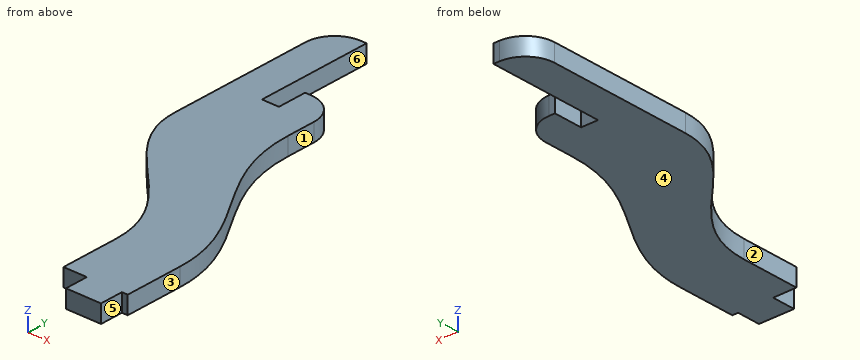
```python
from build123d import *

# Parameters (mm, degrees)
SKETCH1_W           = 6
SKETCH1_H           = 4
BOSS_EXTRUDE1_DEPTH = 3
FILLET1_R           = 5


with BuildPart() as part:
    # Sketch1 → Boss-Extrude1 (new body)
    with BuildSketch(Plane.XY):
        with BuildLine():
            Line((0, 0), (-11, 0))
            Line((-11, 0), (-11, 10))
            add(Edge.make_bspline(
                [(-11, 10), (-11, 23.756315473), (-27.75, 27.611609377), (-27.75, 40)],
                knots=[0, 0, 0, 0, 1, 1, 1, 1], degree=3))
            Line((-27.75, 40), (-27.75, 70))
            Line((-27.75, 70), (-21.75, 70))
            Line((-21.75, 70), (-21.75, 50))
            Line((-21.75, 50), (-18.85, 50))
            Line((-18.85, 50), (-18.85, 55))
            Line((-18.85, 55), (-12.85, 55))
            Line((-12.85, 55), (-12.85, 45))
            add(Edge.make_bspline(
                [(-12.85, 45), (-12.85, 29.868343374), (0, 23.949472312), (0, 10)],
                knots=[0, 0, 0, 0, 1, 1, 1, 1], degree=3))
            Line((0, 10), (0, 0))
        make_face()
        with Locations((-4, -2)):
            Rectangle(SKETCH1_W, SKETCH1_H)
    extrude(amount=BOSS_EXTRUDE1_DEPTH)

    # Fillet1
    fillet1_edges = [part.edges().sort_by_distance(p)[0] for p in [
        (-27.75, 70, 1.5),
        (-12.85, 55, 1.5),
    ]]
    fillet(fillet1_edges, radius=FILLET1_R)


solid = part.part
```
Build history of the part. All positions in model axes, mm. Face numbers are marked on the shaded views. A direction names the side the tool comes from. Round coordinates to 2 decimals unless told otherwise and drop trailing zeros. Write each loop counter-clockwise with the first axis right and the second up, starting at its lowest first coordinate (ties: lowest second). Pieces come first, ordered by that corner, then holes. Notation, with made-up numbers: (66, -19.5) -> (93, -19.5) arc R8 ccw to (93, -10.5) -> close; hole circle Ø5 at (30.25, -13). An arc over 180 degrees is marked (long way). Put each result on its own line as item: value.
Item 1: Wall check: probe 1 along X at (y, z) = (57, 1.1); probe 2 along X at (y, z) = (1.5, 0.3); probe 3 along X at (y, z) = (54, 2.7). Give the ranges that are in metal, low to high. Write a range as from..to.
Here are the results:
probe 1: x = -27.75..-21.75
probe 2: x = -11..0
probe 3: x = -27.75..-21.75, -18.85..-14.85
Item 2: Slice it at A-A, the plane y = 54. Give the cut face in (x, z), plus the area to 3 significant figures.
Here are the results:
outline: (-27.75, 0) -> (-21.75, 0) -> (-21.75, 3) -> (-27.75, 3) -> close; (-18.85, 0) -> (-14.85, 0) -> (-14.85, 3) -> (-18.85, 3) -> close
area: 30.0 mm^2
Item 3: Flat gauge pins, fed straight in: P1, Ø1.5, axis at y = 52.5, z = 0.5, coming from the +X side; P2, Ø1.1, axis at x = -0.5, z = 1, coming from the -Y side; P3, Ø0.5, axis at x = -18.5, z = 1, coming from the +Y side; P4, Ø0.9, axis at y = -3, z = 1.5, coming from the +X side. Where does each tip first touch, or does it go through?
Here are the results:
P1: stops at x = -13.17
P2: stops at y = -4
P3: stops at y = 55
P4: stops at x = -1
Item 4: Slice it at B-B, the plane y = 3.5. Give the cut face in (x, z), plus the area to 3 significant figures.
Here are the results:
outline: (-11, 0) -> (0, 0) -> (0, 3) -> (-11, 3) -> close
area: 33.0 mm^2
Item 5: Tool access for the marked faces 1, 2 and 3: list every direction of +Z, -Z, +X, -X, +Y, -Y with a clear straight run to the whole face (end or side of a thin tool).
Here are the results:
face 1: +Z, -Z, +X, +Y
face 2: +Z, -Z, -X, -Y
face 3: +Z, -Z, +X, +Y, -Y
Item 6: Two-plate mould, pull along X, no slides. Class the marked faces 4, 5 and 6: pulls with the +X half, pulls with the -X half, needs draft (parallel to the pull), parting line crosses it, or undercut.
Here are the results:
face 4: needs draft
face 5: pulls with the +X half
face 6: undercut
